Design review of the part built by this model. Coordinates are the model's own, in mm. A direction names the side the tool comes from. Coordinates: 2 decimals unless noted, no trailing zeros. Order: outer loops, then holes, each group sorted by start corner. A loop starts at its lowest first (then second) coordinate and runs counter-clockwise, first axis right, second up.
from build123d import *

# Parameters (mm, degrees)
HOUSING_BOSS_EXTRUDE1_DEPTH           = 19.3
PLASTIC_SHEILDING_BOSS_EXTRUDE2_DEPTH = 16
SKETCH5_R                             = 2.1
MOUNTING_BRACKETS_BOSS_EXTRUDE3_DEPTH = 0.8
SKETCH6_R                             = 2.5
SHAFT_BOSS_EXTRUDE4_DEPTH             = 15.3
SHAFT_START                           = -11
SHAFT_EDGECUT_EXTRUDE1_DEPTH          = 11
CABLE_HOLE_CUT_EXTRUDE2_DEPTH         = 5


with BuildPart() as part:
    # Sketch2 → Housing Boss-Extrude1 (new body)
    with BuildSketch(Plane.XY):
        with BuildLine():
            Line((-5, -14.198611022), (0, -14.198611022))
            Line((0, -14.198611022), (5, -14.198611022))
            Line((5, -14.198611022), (5, -10.798611022))
            ThreePointArc((5, -10.798611022), (0, 11.9), (-5, -10.798611022))
            Line((-5, -10.798611022), (-5, -14.198611022))
        make_face()
    extrude(amount=-HOUSING_BOSS_EXTRUDE1_DEPTH)

    # Sketch4 → Plastic Sheilding Boss-Extrude2 (add)
    with BuildSketch(Plane.XY):
        with BuildLine():
            Line((0, -16.237711219), (-7, -16.237711219))
            Line((-7, -16.237711219), (-7, -11.151536254))
            Line((-7, -11.151536254), (-7.6, -10.756964563))
            Line((-7.6, -10.756964563), (-7.6, -9.156964563))
            ThreePointArc((-7.6, -9.156964563), (-6.353247262, -10.06211952), (-5, -10.798611022))
            Line((-5, -10.798611022), (-5, -14.198611022))
            Line((-5, -14.198611022), (5, -14.198611022))
            Line((5, -14.198611022), (5, -10.798611022))
            ThreePointArc((5, -10.798611022), (6.353247262, -10.06211952), (7.6, -9.156964563))
            Line((7.6, -9.156964563), (7.6, -10.756964563))
            Line((7.6, -10.756964563), (7, -11.151536254))
            Line((7, -11.151536254), (7, -16.237711219))
            Line((7, -16.237711219), (0, -16.237711219))
        make_face()
    extrude(amount=-PLASTIC_SHEILDING_BOSS_EXTRUDE2_DEPTH)

    # Sketch5 → Mounting Brackets Boss-Extrude3 (add)
    # profile 1 of 2: a face of its own
    with BuildSketch(Plane.XY):
        with BuildLine():
            Line((-15.45, 3.5), (-11.373653766, 3.5))
            ThreePointArc((-11.373653766, 3.5), (-11.9, 0), (-11.373653766, -3.5))
            Line((-11.373653766, -3.5), (-15.45, -3.5))
            ThreePointArc((-15.45, -3.5), (-18.95, 0), (-15.45, 3.5))
        make_face()
        with Locations((-15.45, 0)):
            Circle(SKETCH5_R, mode=Mode.SUBTRACT)
    # profile 2 of 2: a face of its own
    with BuildSketch(Plane.XY):
        with BuildLine():
            Line((15.45, 3.5), (11.373653766, 3.5))
            ThreePointArc((11.373653766, 3.5), (11.9, 0), (11.373653766, -3.5))
            Line((11.373653766, -3.5), (15.45, -3.5))
            ThreePointArc((15.45, -3.5), (18.95, 0), (15.45, 3.5))
        make_face()
        with Locations((15.45, 0)):
            Circle(SKETCH5_R, mode=Mode.SUBTRACT)
    extrude(amount=-MOUNTING_BRACKETS_BOSS_EXTRUDE3_DEPTH)

    # Sketch6 → Shaft Boss-Extrude4 (add)
    with BuildSketch(Plane.XY):
        with Locations((0, 6.5)):
            Circle(SKETCH6_R)
    extrude(amount=SHAFT_BOSS_EXTRUDE4_DEPTH)

    # Sketch7 → Shaft EdgeCut-Extrude1 (cut)
    with BuildSketch(Plane.XY.offset(15.3).offset(SHAFT_START)):
        with BuildLine():
            Line((-2, 8), (2, 8))
            ThreePointArc((2, 8), (0, 9), (-2, 8))
        make_face()
        with BuildLine():
            Line((-2, 5), (2, 5))
            ThreePointArc((2, 5), (0, 4), (-2, 5))
        make_face()
    extrude(amount=SHAFT_EDGECUT_EXTRUDE1_DEPTH, mode=Mode.SUBTRACT)

    # Sketch8 → Cable Hole Cut-Extrude2 (cut)
    with BuildSketch(Plane.XZ.offset(16.237711219)):
        Polygon((0, -2), (3.25, -2), (3.25, -3.2), (0, -3.2), (-3.25, -3.2), (-3.25, -2), align=None)
    extrude(amount=-CABLE_HOLE_CUT_EXTRUDE2_DEPTH, mode=Mode.SUBTRACT)


solid = part.part
1. Add section C-C (z = 12.5). Give the boundary of the cut face in (x, y), and give its area (3 significant figures).
2. Add section A-A (y = 0). Give the boundary of the cut face in (x, z).
3. Add section B-B (x = 0). Give the boundary of the cut face in (y, z), and give its area (3 significant figures).
4. To check wall thickness, follow line 1 (X direction, y = -12.25, z = -3); line 2 (Y direction, x = -15.45, z = -0.55); line 3 (Z direction, x = -3, y = 5.75). State the ranges of each line that lie inside material, in increasing order.
5. Add section D-D (y = 5.5). Give the boundary of the cut face in (x, z).
6. Insertion check: pin 1 (5.5 mm diameter, centred on y = -12.5, z = -6, fed in from +X); pin 2 (5.5 mm diameter, centred on x = 15.45, y = 0, fed in from -Z); pin 3 (12 mm diameter, centred on x = -3, y = -9.5, fed in from +Z); pin 4 (8 mm diameter, centred on x = 9.5, z = 10.5, fed in from +Y). Each pin has a flat end and moves straight along its axis. Give the tip position at first contact, or say it passes through.
7. For faces 4 (the flat face through (-7, -14, -8)), 5 (the flat face through (7, -14, -8)), 6 (the flat face through (0, -14, -3.2)), list the 3-axis set-ups (+Z, -Z, +X, -X, +Y, -Y) from which the entire face can be reached by the end or side of a thin tool; tool diameter is ignored.
8. Mouldability with a two-part tool opening along X and no side actions: class faces 1 (the flat face through (0, -15, -16)), 2 (the flat face through (0, -11.238, -3)), 3 (the flat face through (5, -13, -18)) as pulls with the +X half, pulls with the -X half, needs draft (parallel to the pull), parting line crosses it, or undercut.
Solution:
1. outline: (-2, 5) - (2, 5) arc R2.5 ccw to (2, 8) - (-2, 8) arc R2.5 ccw to start
1. area: 14.0 mm2
2. outline: (-18.95, -0.8) - (-17.55, -0.8) - (-17.55, 0) - (-18.95, 0) - close; (-13.35, -0.8) - (-11.9, -0.8) - (-11.9, -19.3) - (11.9, -19.3) - (11.9, -0.8) - (13.35, -0.8) - (13.35, 0) - (-13.35, 0) - close; (17.55, -0.8) - (18.95, -0.8) - (18.95, 0) - (17.55, 0) - close
3. outline: (-16.24, -16) - (-14.2, -16) - (-14.2, -19.3) - (11.9, -19.3) - (11.9, 0) - (9, 0) - (9, 4.3) - (8, 4.3) - (8, 15.3) - (5, 15.3) - (5, 4.3) - (4, 4.3) - (4, 0) - (-16.24, 0) - (-16.24, -2) - (-11.24, -2) - (-11.24, -3.2) - (-16.24, -3.2) - close
3. area: 585 mm2
4. line 1: x = -7 to -3.25, 3.25 to 7
4. line 2: y = -3.5 to -2.1, 2.1 to 3.5
4. line 3: z = -19.3 to 0
5. outline: (-10.55, -19.3) - (10.55, -19.3) - (10.55, 0) - (2.29, 0) - (2.29, 15.3) - (-2.29, 15.3) - (-2.29, 0) - (-10.55, 0) - close
6. pin 1: stops at x = 7.6
6. pin 2: stops at z = -0.8
6. pin 3: stops at z = 0
6. pin 4: passes through
7. face 4: +Z, -Z, -X, -Y
7. face 5: +Z, -Z, +X, -Y
7. face 6: -Y
8. face 1: needs draft
8. face 2: undercut
8. face 3: pulls with the +X half
